CAD build for the part. Positions are in the model's coordinates, mm. A direction names the side the tool comes from. Give positions to 0.01 mm unless a question says otherwise; leave off trailing zeros. Order: outer loops, then holes, each group sorted by start corner. A loop starts at its lowest first (then second) coordinate and runs counter-clockwise, first axis right, second up.
Item 1: Band-saw the part on A-A on x = 137. Give the cut face in (y, z), plus the area to 3 significant figures.
Item 2: Which spindle directions (+Z, -Z, +X, -X, +Y, -Y) get a long thin tool onto all of the face, cutting with end or side? Do faces 1 (the flat face through (80, 7, 34)), 2 (the cylindrical face through (27.594, 8.783, 12.281)), 3 (the flat face through (55, 15, 40)), 4 (the flat face through (59, 9, 45)). Say none if no direction does.
Item 3: Band-saw the part on B-B on y = 26. Give the cut face in (x, z), plus the area to 3 significant figures.
Item 4: Band-saw the part on C-C on x = 76.5. Give the cut face in (y, z), plus the area to 3 significant figures.
Item 5: Wall check: L1, parallel to Z at x = 19.5, y = 58.5; L2, parallel to X at y = 6, z = 39.5; L3, parallel to X at y = 7.5, z = 47.5. Give the ranges that are in metal, low to high.
Item 6: Flat gauge pins, fed straight in: P1, Ø1.5, axis at x = 42.5, y = 27, coming from the +Z side; P2, Ø4.5, axis at y = 6, z = 38, coming from the -X side; P3, Ø7.5, axis at y = 10.5, z = 33.5, coming from the +X side. Where does each tip first touch, or does it go through?
Item 7: Two-plate mould, pull along Z, no slides. Class faces 5 (the cylindrical face through (82.281, 8.783, 12.406)), 6 (the cylindrical face through (52.14, 12.03, 57.9)), 7 (the flat face through (30, 7, 34)): released by +Z, released by -Z, zero draft, split by the parting line, or undercut.
```python
from build123d import *

# Parameters (mm, degrees)
SKETCH1_W           = 150
SKETCH1_H           = 70
BOSS_EXTRUDE1_DEPTH = 10
BOSS_EXTRUDE2_DEPTH = 15
FILLET1_R           = 8
FILLET2_R           = 8
FILLET3_R           = 8
FILLET4_R           = 8
FILLET5_R           = 8
FILLET6_R           = 8
FILLET11_R          = 8


with BuildPart() as part:
    # Sketch1 → Boss-Extrude1 (new body)
    with BuildSketch(Plane.XY):
        with Locations((75, 35)):
            Rectangle(SKETCH1_W, SKETCH1_H)
    extrude(amount=BOSS_EXTRUDE1_DEPTH)

    # Sketch2 → Boss-Extrude2 (add)
    with BuildSketch(Plane(origin=(0, 0, 0), x_dir=(-1, 0, 0), z_dir=(0, -1, 0))):
        with BuildLine():
            Line((-80, -50), (-80, 0))
            Line((-80, 0), (-30, 0))
            Line((-30, 0), (-30, -50))
            ThreePointArc((-30, -50), (-55, -75), (-80, -50))
        make_face()
    extrude(amount=-BOSS_EXTRUDE2_DEPTH)

    # Fillet1
    fillet1_edges = [part.edges().sort_by_distance(p)[0] for p in [
        (80, 7.5, 10),
    ]]
    fillet(fillet1_edges, radius=FILLET1_R)

    # Fillet2
    fillet2_edges = [part.edges().sort_by_distance(p)[0] for p in [
        (55, 15, 10),
    ]]
    fillet(fillet2_edges, radius=FILLET2_R)

    # Fillet3
    fillet3_edges = [part.edges().sort_by_distance(p)[0] for p in [
        (30, 7.5, 10),
    ]]
    fillet(fillet3_edges, radius=FILLET3_R)

    # Fillet4
    fillet4_edges = [part.edges().sort_by_distance(p)[0] for p in [
        (150, 70, 5),
    ]]
    fillet(fillet4_edges, radius=FILLET4_R)

    # Fillet5
    fillet5_edges = [part.edges().sort_by_distance(p)[0] for p in [
        (150, 0, 5),
    ]]
    fillet(fillet5_edges, radius=FILLET5_R)

    # Fillet6
    fillet6_edges = [part.edges().sort_by_distance(p)[0] for p in [
        (0, 70, 5),
    ]]
    fillet(fillet6_edges, radius=FILLET6_R)

    # Fillet11
    fillet11_edges = [part.edges().sort_by_distance(p)[0] for p in [
        (0, 0, 5),
    ]]
    fillet(fillet11_edges, radius=FILLET11_R)

    # Sketch4 → CBORE for M8 Pan Head Machine Screw1 (revolve, cut)
    with BuildSketch(Plane(origin=(54.842028673, 15, 49.313893032), x_dir=(0, 0, 1), z_dir=(1, 0, 0))):
        Polygon((0, 0), (0, 15), (4.5, 15), (4.5, 6), (9, 6), (9, 0.020977491), (9.025, 0), align=None)
    revolve(axis=Axis((54.842028673, 21.35, 49.313893032), (0, -1, 0)), mode=Mode.SUBTRACT)


solid = part.part
```
The answers:
1. outline: (0, 0) - (70, 0) - (70, 10) - (0, 10) - close
1. area: 700 mm2
2. face 1: +Z, +X, +Y, -Y
2. face 2: +Z, -X, +Y, -Y
2. face 3: +Z, +X, -X, +Y
2. face 4: +Y
3. outline: (0, 0) - (150, 0) - (150, 10) - (0, 10) - close
3. area: 1,500 mm2
4. outline: (0, 0) - (70, 0) - (70, 10) - (23, 10) arc R8 cw to (15, 18) - (15, 62.76) - (0, 62.76) - close
4. area: 1,510 mm2
5. L1: z = 0 to 10
5. L2: x = 30 to 80
5. L3: x = 30 to 50.72, 58.96 to 80
6. P1: stops at z = 10
6. P2: stops at x = 30
6. P3: stops at x = 80
7. face 5: released by +Z
7. face 6: undercut
7. face 7: zero draft
